Geometry check sheet. Reference: the model listing, model coordinates, mm. Give positions to 0.01 mm unless a question says otherwise; leave off trailing zeros. Loops run counter-clockwise (first coordinate to the right, second up) from the corner with the lowest first, then second, coordinate; pieces in that order, holes last. Notation, with made-up numbers: (-36, 32.5) -> (8, 32.5) arc R26 ccw to (8, 60.5) -> close; hole circle Ø3 at (66, 25.5). An arc over 180 degrees is marked (long way). Answer as a JSON object with one key per item and string values.
from build123d import *

# Parameters (mm, degrees)
SKETCH1_R           = 2.2
BOSS_EXTRUDE1_DEPTH = 12


with BuildPart() as part:
    # Sketch1 → Boss-Extrude1 (new body)
    with BuildSketch(Plane(origin=(0, 0, 0), x_dir=(1, 0, 0), z_dir=(0, 1, 0))):
        with BuildLine():
            ThreePointArc((-6.535515489, 3.580947173), (-11.535515489, -1.419052827), (-6.535515489, -6.419052827))
            Line((-6.535515489, -6.419052827), (93.464484511, -6.419052827))
            ThreePointArc((93.464484511, -6.419052827), (98.464484511, -1.419052827), (93.464484511, 3.580947173))
            Line((93.464484511, 3.580947173), (-6.535515489, 3.580947173))
        make_face()
        with Locations((-6.535515489, -1.419052827)):
            Circle(SKETCH1_R, mode=Mode.SUBTRACT)
        with Locations((93.464484511, -1.419052827)):
            Circle(SKETCH1_R, mode=Mode.SUBTRACT)
    extrude(amount=BOSS_EXTRUDE1_DEPTH)


solid = part.part
1) Draft check along Z on faces 1 (the face through (43, 0, 1)), 2 (the face through (43, 6, 6.419)), 3 (the face through (91.267, 5.916, 1.322)), 4 (the face through (-11.534, 5.916, 1.309)). Enter one of: pulls with the +Z half, pulls with the -Z half, needs draft (parallel to the pull), parting line crosses it, or undercut.
Geometry check:
{"face 1": "needs draft", "face 2": "pulls with the +Z half", "face 3": "undercut", "face 4": "parting line crosses it"}
2) Material ranges on line 1 along X through (y, z) = (10.25, 1.5); line 2 along X through (y, z) = (10.25, 3.25); line 3 along X through (y, z) = (8.75, 4.75), recorded low to high. Write a range as from..to.
Geometry check:
{"line 1": "x = -11.53..-8.73, -4.34..91.27, 95.66..98.46", "line 2": "x = -11.19..-7.76, -5.32..92.24, 94.68..98.12", "line 3": "x = -10.26..97.19"}
3) Section check B-B on y = 11. Record the cut outline in (x, z), plus the area to 3 significant figures.
Geometry check:
{"outline": "(-6.54, -3.58) -> (93.46, -3.58) arc R5 ccw to (93.46, 6.42) -> (-6.54, 6.42) arc R5 ccw to start; hole circle Ø4.4 at (-6.54, 1.42); hole circle Ø4.4 at (93.46, 1.42)", "area": "1,050 mm2"}
4) Depth check by flat-ended pin: P1, Ø1, axis at x = 66, z = 1, coming from the -Y side. Enter the tip coordinate at first touch or a pass-through.
Geometry check:
{"P1": "stops at y = 0"}
5) Section check A-A on z = 2.5. Record the cut outline in (x, y).
Geometry check:
{"outline": "(-11.42, 0) -> (-8.45, 0) -> (-8.45, 12) -> (-11.42, 12) -> close; (-4.62, 0) -> (91.55, 0) -> (91.55, 12) -> (-4.62, 12) -> close; (95.38, 0) -> (98.35, 0) -> (98.35, 12) -> (95.38, 12) -> close"}
